from build123d import *

# Parameters (mm, degrees)
BOSS_EXTRUDE1_DEPTH  = 40
SKETCH2_W            = 20
SKETCH2_H            = 20
BOSS_EXTRUDE3_DEPTH  = 20
CUT_EXTRUDE2_DEPTH   = 20
SKETCH5_W            = 20
SKETCH5_H            = 10
CUT_EXTRUDE3_DEPTH   = 20
CUT_EXTRUDE4_DEPTH   = 52
CUT_EXTRUDE8_DEPTH   = 20
BOSS_EXTRUDE11_DEPTH = 20


with BuildPart() as part:
    # Sketch1 → Boss-Extrude1 (new body)
    with BuildSketch(Plane.XY):
        Polygon((20, 20), (0, 20), (0, 0), (40, 0), (40, 40), (20, 40), align=None)
    extrude(amount=BOSS_EXTRUDE1_DEPTH)

    # Sketch2 → Boss-Extrude3 (add)
    with BuildSketch(Plane.ZY.offset(-20)):
        with Locations((10, 30)):
            Rectangle(SKETCH2_W, SKETCH2_H)
    extrude(amount=BOSS_EXTRUDE3_DEPTH)

    # Sketch3 → Cut-Extrude2 (cut)
    with BuildSketch(Plane(origin=(40, 0, 0), x_dir=(0, 0, -1), z_dir=(1, 0, 0))):
        Polygon((0, 0), (-20, 40), (-30, 40), align=None)
        Polygon((0, 40), (-20, 40), (0, 0), align=None)
    extrude(amount=-CUT_EXTRUDE2_DEPTH, mode=Mode.SUBTRACT)

    # Sketch5 → Cut-Extrude3 (cut)
    with BuildSketch(Plane(origin=(0, 0, 0), x_dir=(-1, 0, 0), z_dir=(0, -1, 0))):
        with Locations((-30, -5)):
            Rectangle(SKETCH5_W, SKETCH5_H)
    extrude(amount=-CUT_EXTRUDE3_DEPTH, mode=Mode.SUBTRACT)

    # Sketch6 → Cut-Extrude4 (cut)
    with BuildSketch(Plane.XZ):
        Polygon((20, 0), (0, 20), (0, 0), align=None)
    extrude(amount=-CUT_EXTRUDE4_DEPTH, mode=Mode.SUBTRACT)

    # Sketch7 → Cut-Extrude8 (cut)
    with BuildSketch(Plane(origin=(40, 0, 0), x_dir=(0, 0, -1), z_dir=(1, 0, 0))):
        Polygon((-10, 0), (-30, 40), (-10, 13.333333333), align=None)
    extrude(amount=-CUT_EXTRUDE8_DEPTH, mode=Mode.SUBTRACT)

    # Sketch14 → Boss-Extrude11 (add)
    with BuildSketch(Plane(origin=(0, 40, 0), x_dir=(1, 0, 0), z_dir=(0, 1, 0))):
        Polygon((0, -20), (20, -40), (20, -20), align=None)
    extrude(amount=-BOSS_EXTRUDE11_DEPTH)


solid = part.part
Input: part model. Units: mm. Frame: model coordinates. A direction names the side the tool comes from. Coordinates: 2 decimals unless noted, no trailing zeros. Loops run counter-clockwise (first coordinate to the right, second up) from the corner with the lowest first, then second, coordinate; pieces in that order, holes last. Notation, with made-up numbers: (-22, 71.25) -> (28, 71.25) arc R31 cw to (28, 100.25) -> close; hole circle Ø8 at (47.5, 62). An arc over 180 degrees is marked (long way). Write each question's results on one line, items separated by ' | '. Start each with the question number.
Q1. Section A-A, the plane x = 9.5. Return the cut outline in (y, z).
Q2. Section D-D, the plane x = 30. Return the cut outline in (y, z), plus the area to 3 significant figures.
Q3. Section C-C, the plane z = 25. Return the cut outline in (x, y), plus the area to 3 significant figures.
Q4. Ray query, line 1 (Z direction, x = 32.5, y = 20); line 2 (Y direction, x = 8, z = 37.5); line 3 (Z direction, x = 2.5, y = 10.5). Return the intervals inside material, ascending. Write a range as from..to.
Q5. Pin query (flat end, axial travel): pin 1 (5 mm diameter, centred on x = 36, y = 12.5, fed in from -Z); pin 2 (10 mm diameter, centred on y = 34, z = 18.5, fed in from -X); pin 3 (4 mm diameter, centred on y = 14.5, z = 6, fed in from +X); pin 4 (6 mm diameter, centred on x = 16.5, y = 34.5, fed in from +Z). Return the tip coordinate at first contact, or that it passes through.
Q6. Reachability of faces 1 (the flat face through (24, 16, 40)), 2 (the flat face through (10, 30, 30)), 3 (the flat face through (30, 20, 20)) from +Z, -Z, +X, -X, +Y, -Y: full face, straight path, thin tool, end or side. Return the list, or none.
Q7. Section B-B, the plane z = 34. Return the cut outline in (x, y).
Found:
1) outline: (0, 10.5) -> (40, 10.5) -> (40, 29.5) -> (20, 29.5) -> (20, 40) -> (0, 40) -> close
2) outline: (0, 10) -> (40, 30) -> (40, 40) -> (0, 40) -> close | area: 800 mm2
3) outline: (0, 0) -> (40, 0) -> (40, 30) -> (20, 30) -> (20, 40) -> (5, 40) -> (5, 20) -> (0, 20) -> close | area: 1,300 mm2
4) line 1: 20..40 | line 2: 0..20 | line 3: 17.5..40
5) pin 1: z = 15 | pin 2: x = 0 | pin 3: x = 20 | pin 4: z = 39.5
6) face 1: +Z, +X, -X, +Y, -Y | face 2: +Z, -X, +Y | face 3: -Z, +X, +Y
7) outline: (0, 0) -> (40, 0) -> (40, 40) -> (14, 40) -> (14, 20) -> (0, 20) -> close
